Verification items for the finished model (mm, model axes). Round coordinates to 2 decimals unless told otherwise and drop trailing zeros. Order: outer loops, then holes, each group sorted by start corner. A loop starts at its lowest first (then second) coordinate and runs counter-clockwise, first axis right, second up. Notation, with made-up numbers: M 49.25,24 L 86.25,24 A26 cw 86.25,59 Z; hole C 46,39 d6. An arc over 180 degrees is marked long. Answer as a JSON object with one key per item and string values. Group by question number.
```python
from build123d import *

# Parameters (mm, degrees)
F0_W     = 50.8
F0_H     = 101.6
F0_R     = 7.62
F1_DEPTH = 12.7
F2_R     = 5.08
F3_R     = 3.515063
F4_DEPTH = 25.4


with BuildPart() as f1:
    # F0 (on Front) → F1 (new body, symmetric)
    with BuildSketch(Plane.XZ):
        Rectangle(F0_W, F0_H)
        with Locations((0, -33.737253)):
            Circle(F0_R, mode=Mode.SUBTRACT)
        with Locations((0, 33.737253)):
            Circle(F0_R, mode=Mode.SUBTRACT)
    extrude(amount=F1_DEPTH, both=True)

    # F2
    f2_edges = [f1.edges().sort_by_distance(p)[0] for p in [
        (25.4, 0, -50.8),
        (-25.4, 0, -50.8),
        (25.4, 0, 50.8),
        (-25.4, 0, 50.8),
    ]]
    fillet(f2_edges, radius=F2_R)

    # F3 (on face) → F4 (cut, symmetric)
    with BuildSketch(Plane.XZ.offset(12.7)):
        with Locations((-20.32, 45.72)):
            Circle(F3_R)
        with Locations((-20.32, -45.72)):
            Circle(F3_R)
        with Locations((20.32, 45.72)):
            Circle(F3_R)
        with Locations((20.32, -45.72)):
            Circle(F3_R)
    extrude(amount=F4_DEPTH, both=True, mode=Mode.SUBTRACT)


solid = f1.part
```
Q1. Release check for a two-part mould opening along Z. For faces 1 (the face through (-25.4, 0, -1)), 2 (the face through (-16.97, -0.18, 46.78)), 3 (the face through (0, 0, 50.8)) record: released by +Z, released by -Z, zero draft, split by the parting line, or undercut.
Q2. Cross-section at C-C, the plane y = 8.75. Record the cut outline in (x, z), then the cut area to 3 significant figures.
Q3. Cross-section at A-A, the plane x = 0. Record the cut outline in (y, z), then the cut area to 3 significant figures.
Q4. Gauge pin test, flat end, axial feed: pin 1 Ø5.5 at (x, z) = (20.32, 45.72) entering from -Y. Record the tip position at first contact, or that the pin passes through.
Q5. Thickness scan on line 1 (Z direction, x = 20.32, y = 2.5); line 2 (Z direction, x = 0, y = -4.25); line 3 (X direction, y = 2.75, z = 34). Record the ranges inside material, lowest first. Write a range as from..to.
Q6. Cross-section at B-B, the plane z = 38. Record the cut outline in (x, y).
Q7. Cross-section at D-D, the plane x = 21.5. Record the cut outline in (y, z).
Conclusion:
{
 "1": {"face 1": "zero draft", "face 2": "undercut", "face 3": "released by +Z"},
 "2": {"outline": "M -25.4,-45.72 A5.08 ccw -20.32,-50.8 L 20.32,-50.8 A5.08 ccw 25.4,-45.72 L 25.4,45.72 A5.08 ccw 20.32,50.8 L -20.32,50.8 A5.08 ccw -25.4,45.72 Z; hole C -20.32,-45.72 d7.03; hole C -20.32,45.72 d7.03; hole C 0,-33.74 d15.24; hole C 0,33.74 d15.24; hole C 20.32,-45.72 d7.03; hole C 20.32,45.72 d7.03", "area": "4,620 mm2"},
 "3": {"outline": "M -12.7,-50.8 L 12.7,-50.8 L 12.7,-41.36 L -12.7,-41.36 Z; M -12.7,-26.12 L 12.7,-26.12 L 12.7,26.12 L -12.7,26.12 Z; M -12.7,41.36 L 12.7,41.36 L 12.7,50.8 L -12.7,50.8 Z", "area": "1,810 mm2"},
 "4": {"pin 1": "through"},
 "5": {"line 1": "-50.8..-49.24, -42.2..42.2, 49.24..50.8", "line 2": "-50.8..-41.36, -26.12..26.12, 41.36..50.8", "line 3": "-25.4..-7.62, 7.62..25.4"},
 "6": {"outline": "M -25.4,-12.7 L -6.32,-12.7 L -6.32,12.7 L -25.4,12.7 Z; M 6.32,-12.7 L 25.4,-12.7 L 25.4,12.7 L 6.32,12.7 Z"},
 "7": {"outline": "M -12.7,-50.66 L 12.7,-50.66 L 12.7,-49.03 L -12.7,-49.03 Z; M -12.7,-42.41 L 12.7,-42.41 L 12.7,42.41 L -12.7,42.41 Z; M -12.7,49.03 L 12.7,49.03 L 12.7,50.66 L -12.7,50.66 Z"}
}
